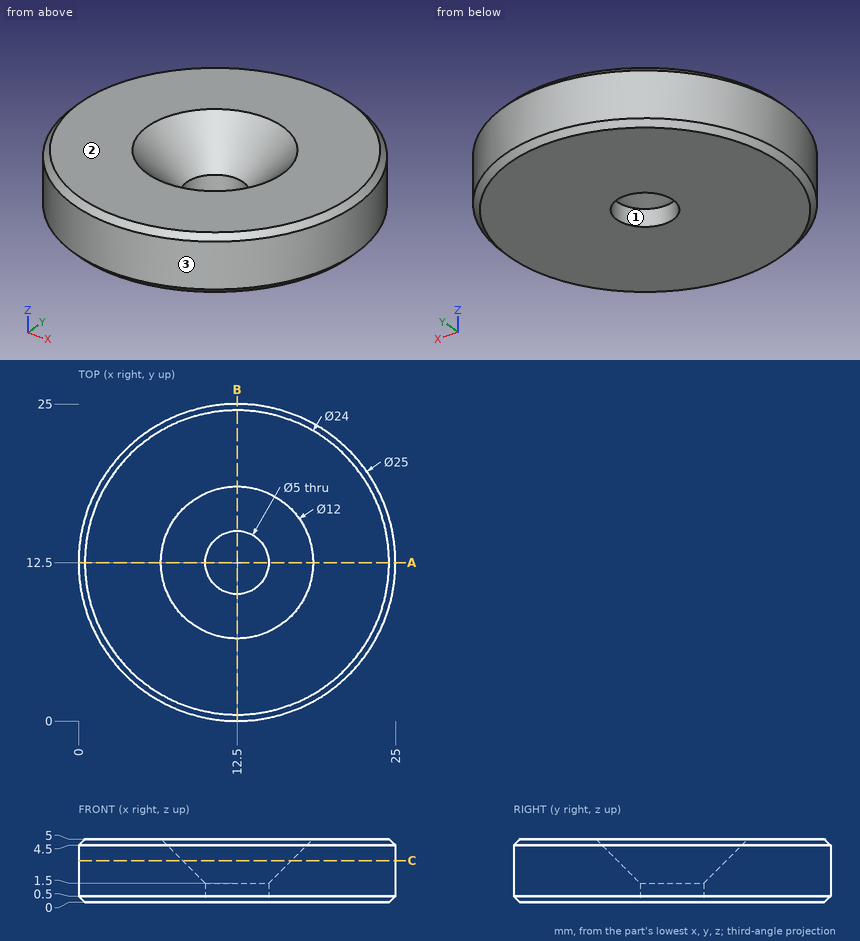
Design review of the part shown in the three views and the two pictorial views. Dimensions are in mm from the part's minimum x, y and z. Round coordinates to 2 decimals unless told otherwise and drop trailing zeros. Write each loop counter-clockwise with the first axis right and the second up, starting at its lowest first coordinate (ties: lowest second). Pieces come first, ordered by that corner, then holes.
Item 1: For pin 1 Ø1 at (y, z) = (18, 0.5) entering from -X; pin 2 Ø4.5 at (x, y) = (12.5, 12.5) entering from +Z; pin 3 Ø3 at (x, z) = (7, 4.5) entering from +Y; pin 4 Ø1.5 at (x, z) = (7, 2.5) entering from -Y, all flat-tipped, find the tip position at first contact; note any pin that passes through.
Item 2: Consider section A-A on y = 12.5. Give the boundary of the cut face in (x, z), and give its area (4 significant figures).
Item 3: Draft analysis for pull direction X (two halves, no side actions). For the marked faces 1, 2 and 3, state which applies: released by +X, released by -X, zero draft, split by the parting line, or undercut.
Item 4: Wall thickness on L1, parallel to Y at x = 12.5, z = 0.9; L2, parallel to Y at x = 16.25, z = 3.65; L3, parallel to X at y = 10.5, z = 1.1: over which ranges is each line inside the solid? List them lowest first.
Item 5: Consider section C-C on z = 3.3. Give the boundary of the cut face in (x, y), and give its area (3 significant figures).
Check values:
1. pin 1: stops at x = 1.04
1. pin 2: passes through
1. pin 3: stops at y = 24.34
1. pin 4: stops at y = 0.94
2. outline: (0, 0.5) - (0.5, 0) - (10, 0) - (10, 1.5) - (6.5, 5) - (0.5, 5) - (0, 4.5) - close; (15, 0) - (24.5, 0) - (25, 0.5) - (25, 4.5) - (24.5, 5) - (18.5, 5) - (15, 1.5) - close
2. area: 87.25 mm2
3. face 1: undercut
3. face 2: zero draft
3. face 3: split by the parting line
4. L1: y = 0 to 10, 15 to 25
4. L2: y = 0.58 to 9.75, 15.25 to 24.42
4. L3: x = 0.16 to 11, 14 to 24.84
5. outline: circle Ø25 at (12.5, 12.5); hole circle Ø8.6 at (12.5, 12.5)
5. area: 433 mm2
